from build123d import *

# Parameters (mm, degrees)
F1_W     = 17.993393
F1_H     = 34.332218
F2_ANGLE = -180


with BuildPart() as f2:
    # F1 (on face) → F2 (revolve)
    with BuildSketch(Plane.XY):
        Polygon((12.023137, 4.216103), (-5.970256, 4.216103), (-5.970256, -13.156827), (47.803093, -13.156827), (47.803093, 4.216103), align=None)
        with Locations((3.026441, 21.382212)):
            Rectangle(F1_W, F1_H)
    revolve(axis=Axis((24.225553, -28.875191, 0), (-1, 0, 0)), revolution_arc=F2_ANGLE)

    # F1 (on face) → F3 (revolve)
    with BuildSketch(Plane.XY):
        Polygon((54.421362, 26.139084), (54.421362, -13.156827), (54.421362, -28.875191), (65.176025, -28.875191), (65.176025, 26.139084), align=None)
        Polygon((19.468673, 26.139084), (54.421362, 26.139084), (65.176025, 26.139084), (65.176025, 35.032369), (19.468673, 35.032369), align=None)
        Polygon((47.803093, -13.156827), (-5.970256, -13.156827), (-5.970256, -28.875191), (54.421362, -28.875191), (54.421362, -13.156827), align=None)
    revolve(axis=Axis((59.798693, -28.875191, 0), (-1, 0, 0)))


solid = f2.part
Work out the finished part from the listing and answer in its coordinate system (mm). A direction names the side the tool comes from. Coordinates: 2 decimals unless noted, no trailing zeros. Write each loop counter-clockwise with the first axis right and the second up, starting at its lowest first coordinate (ties: lowest second). Pieces come first, ordered by that corner, then holes. Notation, with made-up numbers: (12.25, 61.5) - (31.25, 61.5) arc R10 ccw to (31.25, 78.5) - close; hole circle Ø2 at (67, 83.5). An arc over 180 degrees is marked (long way). One line per question, with ' | ' between items.
1) The mould has two halves that part along X. Classify faces 6 (the face through (42, 5.48, -53.89)), 7 (the face through (65.176, -28, -1)), 8 (the face through (-5.97, -29, 8)), 9 (the face through (19.469, -1, -48)): +X half, -X half, draft (parallel to the pull), parting line (faces both ways), or undercut.
Checks:
face 6: draft | face 7: +X half | face 8: -X half | face 9: undercut
2) Consider probe 1 along X at (y, z) = (-2.5, 2); probe 2 along X at (y, z) = (-63.5, 47.5); probe 3 along Z at (x, y) = (46, -3). Determine where each line is inside the solid, lowest interval first. Write a range as [from, to].
Checks:
probe 1: [-5.97, 47.8], [54.42, 65.18] | probe 2: [-5.97, 12.02], [19.47, 65.18] | probe 3: [-58.44, -48.55], [0, 20.63], [48.55, 58.44]
3) Find section A-A, the plane y = -56. Determine the outline of the cut face in (x, z), and give its area (3 significant figures).
Checks:
outline: (-5.97, 0) - (47.8, 0) - (47.8, 18.95) - (12.02, 18.95) - (12.02, 61.73) - (-5.97, 61.73) - close; (19.47, -57.87) - (65.18, -57.87) - (65.18, 57.87) - (19.47, 57.87) - (19.47, 47.86) - (54.42, 47.86) - (54.42, -47.86) - (19.47, -47.86) - close | area: 3,730 mm2
4) Flat-ended cylindrical pins translate along their axes: P1, Ø1.5, axis at y = -69.5, z = -45, coming from the -X side; P2, Ø1, axis at x = 48.5, y = -42, coming from the -Z side; P3, Ø8, axis at x = 28, y = 19, coming from the +Z side. Find the tip coordinate at first contact, or state that the pin passes through.
Checks:
P1: x = 19.47 | P2: z = -62.65 | P3: z = 46.47
5) For faces 1 (the face through (-5.97, -28, 34)), 2 (the face through (15, -59, 0)), 3 (the face through (12.023, -28, 34)), 4 (the face through (47.803, -28, 17)), 5 (the face through (3.152, -27.393, 67.407)), determine the directions among +Z, -Z, +X, -X, +Y, -Y from which every point of the face is accessible in a straight line to the end or side of a thin tool.
Checks:
face 1: +Z, -Z, -X, +Y, -Y | face 2: -X | face 3: +Z | face 4: none | face 5: +Z, +X, -X
6) Find section B-B, the plane z = 31. Determine the outline of the cut face in (x, y), and give its area (3 significant figures).
Checks:
outline: (-5.97, -88.75) - (12.02, -88.75) - (12.02, -40.45) - (47.8, -40.45) - (47.8, -17.3) - (12.02, -17.3) - (12.02, 31) - (-5.97, 31) - close; (19.47, -84.76) - (65.18, -84.76) - (65.18, 27.01) - (19.47, 27.01) - (19.47, 16.57) - (54.42, 16.57) - (54.42, -74.32) - (19.47, -74.32) - close | area: 4,910 mm2
7) Find section D-D, the plane y = -22. Determine the outline of the cut face in (x, z), and give its area (3 significant figures).
Checks:
outline: (-5.97, -14.14) - (54.42, -14.14) - (54.42, -54.58) - (19.47, -54.58) - (19.47, -63.54) - (65.18, -63.54) - (65.18, 63.54) - (19.47, 63.54) - (19.47, 54.58) - (54.42, 54.58) - (54.42, 14.14) - (47.8, 14.14) - (47.8, 32.37) - (12.02, 32.37) - (12.02, 67.07) - (-5.97, 67.07) - close | area: 5,300 mm2
8) Find section C-C, the plane z = 9. Determine the outline of the cut face in (x, y), and give its area (3 significant figures).
Checks:
outline: (-5.97, -95.7) - (12.02, -95.7) - (12.02, -60.72) - (47.8, -60.72) - (47.8, -41.76) - (54.42, -41.76) - (54.42, -83.15) - (19.47, -83.15) - (19.47, -92.15) - (65.18, -92.15) - (65.18, 34.4) - (19.47, 34.4) - (19.47, 25.4) - (54.42, 25.4) - (54.42, -15.99) - (47.8, -15.99) - (47.8, 2.97) - (12.02, 2.97) - (12.02, 37.94) - (-5.97, 37.94) - close | area: 6,840 mm2
